Can you work these out from the model? Positions are in its coordinate system, mm. A direction names the side the tool comes from. Give positions to 0.01 mm unless a question says otherwise; leave off trailing zeros. Order: outer loops, then holes, each group sorted by start corner. A loop starts at its lowest first (then second) coordinate and runs counter-clockwise, first axis right, second up. Notation, with made-up numbers: (-7, -31) - (52, -31) arc R7 ccw to (52, -23) - close; hole circle Ø3 at (25.5, 72.5). An arc over 180 degrees is marked (long way). Write each question's results on one line, items separated by ' | '. Start each with the question number.
from build123d import *

# Parameters (mm, degrees)
BOSS_EXTRUDE1_DEPTH                                  = 53
CSK_FOR_M2_5_COUNTERSUNK_FLAT_HEAD_SCREW_D           = 2.9
CSK_FOR_M2_5_COUNTERSUNK_FLAT_HEAD_SCREW_DEPTH       = 14
CSK_FOR_M2_5_COUNTERSUNK_FLAT_HEAD_SCREW_CSINK_D     = 5.5
CSK_FOR_M2_5_COUNTERSUNK_FLAT_HEAD_SCREW_CSINK_ANGLE = 90
CSK_FOR_M2_5_COUNTERSUNK_FLAT_HEAD_SCREW_TIP         = 0.871247898
BOSS_EXTRUDE2_DEPTH                                  = 2.2


with BuildPart() as part:
    # Sketch1 → Boss-Extrude1 (new body)
    with BuildSketch(Plane(origin=(0, 0, 0), x_dir=(0, 0, -1), z_dir=(1, 0, 0))):
        Polygon((4, 0.5), (6, 0.5), (6, -2.5), (-6, -2.5), (-6, 0.5), (-4, 0.5), (-4, 1.5), (-7, 1.5), (-7, 2.5), (7, 2.5), (7, 1.5), (4, 1.5), align=None)
    extrude(amount=BOSS_EXTRUDE1_DEPTH)

    # CSK for M2.5 Countersunk Flat Head Screw1
    with Locations(Plane(origin=(42, 2.5, 0.10398467), x_dir=(0, 0, 1), z_dir=(0, 1, 0))):
        with Locations((0, 0)):
            CounterSinkHole(CSK_FOR_M2_5_COUNTERSUNK_FLAT_HEAD_SCREW_D / 2, CSK_FOR_M2_5_COUNTERSUNK_FLAT_HEAD_SCREW_CSINK_D / 2, depth=CSK_FOR_M2_5_COUNTERSUNK_FLAT_HEAD_SCREW_DEPTH, counter_sink_angle=CSK_FOR_M2_5_COUNTERSUNK_FLAT_HEAD_SCREW_CSINK_ANGLE)
            with Locations((0, 0, -(CSK_FOR_M2_5_COUNTERSUNK_FLAT_HEAD_SCREW_DEPTH + CSK_FOR_M2_5_COUNTERSUNK_FLAT_HEAD_SCREW_TIP / 2))):  # 118° drill point
                Cone(0, CSK_FOR_M2_5_COUNTERSUNK_FLAT_HEAD_SCREW_D / 2, CSK_FOR_M2_5_COUNTERSUNK_FLAT_HEAD_SCREW_TIP, mode=Mode.SUBTRACT)

    # Sketch2 → Boss-Extrude2 (add)
    with BuildSketch(Plane(origin=(0, 2.5, 0), x_dir=(1, 0, 0), z_dir=(0, 1, 0))):
        with BuildLine():
            ThreePointArc((14.15, -0.10398467), (11, 3.04601533), (7.85, -0.10398467))
            ThreePointArc((7.85, -0.10398467), (11, -3.25398467), (14.15, -0.10398467))
        make_face()
        with BuildLine():
            ThreePointArc((31.15, -0.10398467), (28, 3.04601533), (24.85, -0.10398467))
            ThreePointArc((24.85, -0.10398467), (28, -3.25398467), (31.15, -0.10398467))
        make_face()
    extrude(amount=BOSS_EXTRUDE2_DEPTH)


solid = part.part
Q1. Which directions (+Z, -Z, +X, -X, +Y, -Y) give clear straight access to the entire face, cutting with the end or side of a thin tool? Please do faces 5 (the flat face through (26, 1.5, 5)), 6 (the flat face through (26, -1, -6)), 7 (the flat face through (26, 0.5, -5)).
Q2. If we section it at A-A (z = 4.5): Please give me the cut outline in (x, y).
Q3. Will these pins go through, and if not, where does the flat tip stop? P1, Ø1, axis at x = 18.5, z = -5.5, coming from the +Y side; P2, Ø2.5, axis at x = 34, y = -1.5, coming from the +Z side; P3, Ø3.5, axis at x = 32.5, y = -0.5, coming from the -Z side.
Q4. If we section it at D-D (x = 28): Please give me the cut outline in (y, z), plus the area to 3 significant figures.
Q5. Thinking about a two-plate mould opening in Z: for faces 1 (the flat face through (26, 1, 4)), 2 (the flat face through (26, 1, -4)), 3 (the cylindrical face through (40.714, -0.676, -0.565)), 4 (the flat face through (26, 2.5, 3)), which applies, released by +Z, released by -Z, zero draft, split by the parting line, or undercut?
Q6. If we section it at B-B (x = 42): Please give me the cut outline in (y, z).
Q7. If we section it at C-C (y = -1): Please give me the cut outline in (x, z).
Q8. If I drill on probe 1 along Z at (x, y) = (42, 0.45); probe 2 along Y at (x, z) = (26.5, -4.75); probe 3 along X at (y, z) = (-1.25, 0), over which ranges is the centre line in solid material (lowest first)? Write a range as from..to.
Findings below:
1) face 5: +Z, +X, -X | face 6: -Z, +X, -X, -Y | face 7: -Z, +X, -X
2) outline: (0, -2.5) - (53, -2.5) - (53, 0.5) - (0, 0.5) - close; (0, 1.5) - (53, 1.5) - (53, 2.5) - (0, 2.5) - close
3) P1: stops at y = 2.5 | P2: stops at z = 6 | P3: stops at z = -6
4) outline: (-2.5, -6) - (0.5, -6) - (0.5, -4) - (1.5, -4) - (1.5, -7) - (2.5, -7) - (2.5, -3.05) - (4.7, -3.05) - (4.7, 3.25) - (2.5, 3.25) - (2.5, 7) - (1.5, 7) - (1.5, 4) - (0.5, 4) - (0.5, 6) - (-2.5, 6) - close | area: 71.9 mm2
5) face 1: released by +Z | face 2: released by -Z | face 3: undercut | face 4: zero draft
6) outline: (-2.5, -6) - (0.5, -6) - (0.5, -4) - (1.5, -4) - (1.5, -7) - (2.5, -7) - (2.5, -2.65) - (1.2, -1.35) - (-2.5, -1.35) - close; (-2.5, 1.55) - (1.2, 1.55) - (2.5, 2.85) - (2.5, 7) - (1.5, 7) - (1.5, 4) - (0.5, 4) - (0.5, 6) - (-2.5, 6) - close
7) outline: (0, -6) - (53, -6) - (53, 6) - (0, 6) - close; hole circle Ø2.9 at (42, 0.1)
8) probe 1: z = -6..-1.35, 1.55..6 | probe 2: y = -2.5..0.5, 1.5..2.5 | probe 3: x = 0..40.55, 43.45..53
